from build123d import *

# Parameters (mm, degrees)
F_1_4_0_5_DIAMETER_HOLE2_D = 12.7


with BuildPart() as part:
    # Sketch1 → Revolve3 (revolve)
    with BuildSketch(Plane(origin=(0, 0, 0), x_dir=(0, 0, -1), z_dir=(1, 0, 0))):
        Polygon((-38.1, 0), (-38.1, 22.098), (-34.925, 22.098), (-34.925, 4.826), (-9.525, 4.826), (-5.198570671, 29.3624), (0, 29.3624), (0, -29.3624), (-5.198570671, -29.3624), (-9.525, -4.826), (-34.925, -4.826), (-34.925, -22.352), (-38.1, -22.352), align=None)
    revolve(axis=Axis((0, 29.3624, -12.7), (0, -1, 0)))

    # 1/4 (0.5) Diameter Hole2 (through all)
    with Locations(Plane(origin=(0, 4.826, 0), x_dir=(1, 0, 0), z_dir=(0, 1, 0))):
        with Locations((-17.4625, 42.945937227), (17.4625, 42.945937227), (34.91559931, 11.889722379), (17.4625, -17.545937227), (-17.4625, -17.545937227), (-34.916879179, 11.946890841)):
            Hole(F_1_4_0_5_DIAMETER_HOLE2_D / 2)


solid = part.part
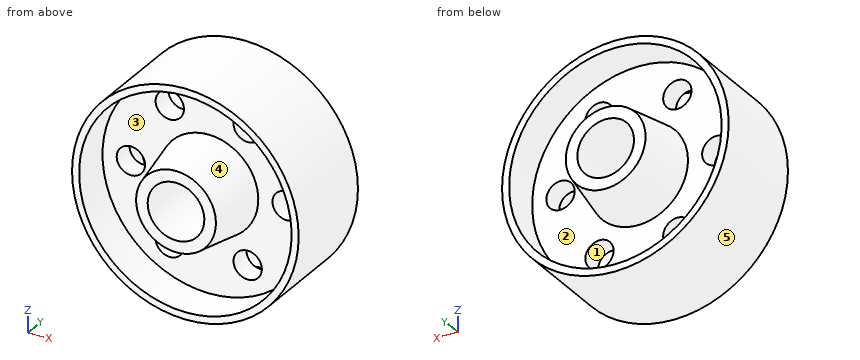
Build history of the part. All positions in model axes, mm. Face numbers are marked on the shaded views. A direction names the side the tool comes from. Give positions to 0.01 mm unless a question says otherwise; leave off trailing zeros. Order: outer loops, then holes, each group sorted by start corner. A loop starts at its lowest first (then second) coordinate and runs counter-clockwise, first axis right, second up. Notation, with made-up numbers: M 83,-29 L 87,-29 A15 cw 87,-6 Z; hole C -25.5,-36.75 d3. An arc over 180 degrees is marked long. Use one line per item in the form item = value.
Q1. Slice it at C-C, the plane y = 20. Write the cut outline in (x, z) (3 decimals), and give its area (3 significant figures).
Conclusion:
outline = C 0,-12.7 d101.6; C 0,-12.7 d39.099; hole C 0,-12.7 d95.25; hole C 0,-12.7 d25.4
area = 1,680 mm2
Q2. Which spindle directions (+Z, -Z, +X, -X, +Y, -Y) get a long thin tool onto all of the face, cutting with end or side? Do the marked faces 1, 2 and 3. Say none if no direction does.
Conclusion:
face_1 = +Y, -Y
face_2 = +Y
face_3 = -Y
Q3. Pull direction Z, two halves, no side cores. Call the marked faces 4 and 5: released by +Z, released by -Z, zero draft, split by the parting line, or undercut.
Conclusion:
face_4 = undercut
face_5 = split by the parting line
Q4. Slice it at B-B, the plane z = 14.5. Write the cut outline in (x, y), and give its area (3 significant figures).
Conclusion:
outline = M -42.9,-22.35 L -39.09,-22.35 L -39.09,-4.83 L -23.03,-4.83 L -23.03,4.83 L -39.09,4.83 L -39.09,22.1 L -42.9,22.1 Z; M -11.89,-4.83 L 11.89,-4.83 L 11.89,4.83 L -11.89,4.83 Z; M 23.03,-4.83 L 39.09,-4.83 L 39.09,-22.35 L 42.9,-22.35 L 42.9,22.1 L 39.09,22.1 L 39.09,4.83 L 23.03,4.83 Z
area = 878 mm2
Q5. Wall check: probe 1 along X at (y, z) = (2.5, 17); probe 2 along X at (y, z) = (-5.5, -29.5); probe 3 along X at (y, z) = (6, -20). Give the ranges that are in metal, low to high.
Conclusion:
probe_1 = -41.21 to -23.79, -11.14 to 11.14, 23.79 to 41.21
probe_2 = -47.94 to -44.56, -14.37 to 14.37, 44.56 to 47.94
probe_3 = -50.27 to -47.06, -20.77 to -10.39, 10.39 to 20.77, 47.06 to 50.27
Q6. Slice it at D-D, the plane x = 32.5. Write the cut outline in (y, z), and give its area (3 significant figures).
Conclusion:
outline = M -22.35,-51.74 L 22.1,-51.74 L 22.1,-47.51 L 4.83,-47.51 L 4.83,-17.76 L -4.83,-17.76 L -4.83,-47.51 L -22.35,-47.51 Z; M -22.35,22.11 L -4.83,22.11 L -4.83,-6.02 L 4.83,-6.02 L 4.83,22.11 L 22.1,22.11 L 22.1,26.34 L -22.35,26.34 Z
area = 935 mm2
Q7. Slice it at A-A, the plane x = 0. Write the cut outline in (y, z) (3 decimals), and give its area (3 significant figures).
Conclusion:
outline = M -29.362,-30.599 L -4.826,-34.925 L -4.826,-60.325 L -22.352,-60.325 L -22.352,-63.5 L 22.098,-63.5 L 22.098,-60.325 L 4.826,-60.325 L 4.826,-34.925 L 29.362,-30.599 L 29.362,-25.4 L -29.362,-25.4 Z; M -29.362,0 L 29.362,0 L 29.362,5.199 L 4.826,9.525 L 4.826,34.925 L 22.098,34.925 L 22.098,38.1 L -22.352,38.1 L -22.352,34.925 L -4.826,34.925 L -4.826,9.525 L -29.362,5.199 Z
area = 1,680 mm2
Q8. Pin check, flat tips, straight feed: P1, Ø14.5, axis at x = 17.46, z = 17.55, coming from the +Y side; P2, Ø6, axis at y = -19, z = 1, coming from the -X side; P3, Ø1, axis at x = 25.5, y = 19.5, coming from the +Z side. Stop position of each tip, or through.
Conclusion:
P1 = 4.83
P2 = -49.66
P3 = 31.52
